Autodesk Inventor part; units mm, degrees
ref_plane "YZ Plane" through (0, 0, 0) normal (1, 0, 0) x (0, 1, 0)
ref_plane "XZ Plane" through (0, 0, 0) normal (0, 1, 0) x (-1, 0, 0)
ref_plane "XY Plane" through (0, 0, 0) normal (0, 0, 1) x (1, 0, 0)
sketch "Sketch2" plane through (0, 0, 0) normal (1, 0, 0) x (0, 1, 0)
  circle A0 centre (0, 0) radius 21.5
  dimension "d3" = 43
extrude "Extrusion1" add sketch "Sketch2" along normal blind 2
sketch "Sketch3" plane through (2, 0, 0) normal (1, 0, 0) x (0, 0, -1)
  circle A0 centre (0, 0) radius 21.5
  circle A1 centre (0, 0) radius 8.5
  dimension "d6" = 17
extrude "Extrusion2" cut sketch "Sketch3" against normal blind 2 contours A1
sketch "Sketch4" plane through (2, 0, 0) normal (1, 0, 0) x (0, 0, -1)
  circle A0 centre (0, 0) radius 8.5
  circle A1 centre (0, 0) radius 21.5
  circle A2 centre (0, 0) radius 9.5
  dimension "d9" = 19
extrude "Extrusion3" add sketch "Sketch4" along normal blind 7 contours A2
properties part number "holeCoverP2"
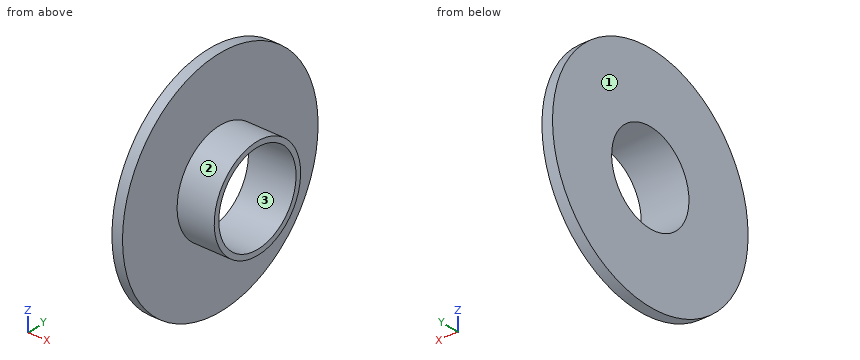
Read the model definition and answer for the solid it produces. Units are mm, in the model's axes. Face numbers are marked on the shaded views. Give positions to 0.01 mm unless a question says otherwise; leave off trailing zeros. Write each loop counter-clockwise with the first axis right and the second up, starting at its lowest first coordinate (ties: lowest second). Pieces come first, ordered by that corner, then holes. Notation, with made-up numbers: (50, -15) -> (87, -15) arc R35 ccw to (87, 20) -> close; hole circle Ø6 at (-4, -34). An arc over 180 degrees is marked (long way). Answer in a Markdown table with one row per item.
1) Straight lines are drawn through the part: line 1 (Y direction, x = 2.25, z = 0); line 2 (X direction, y = -10.5, z = 7); line 3 (Y direction, x = 6.5, z = 1). For each, find the intervals that lie inside material, in ascending order. Write a range as [from, to].
Results list:
| item | result |
|---|---|
| line 1 | [-9.5, -8.5], [8.5, 9.5] |
| line 2 | [0, 2] |
| line 3 | [-9.45, -8.44], [8.44, 9.45] |
2) Section D-D on z = -9 is taken. Give the vertices of the cut face in (x, y), plus the area to 3 significant figures.
Results list:
| item | result |
|---|---|
| outline | (0, -19.53) -> (2, -19.53) -> (2, -3.04) -> (9, -3.04) -> (9, 3.04) -> (2, 3.04) -> (2, 19.53) -> (0, 19.53) -> close |
| area | 121 mm^2 |
3) Each of these flat-tipped pins is pushed along its axis until it touches: pin 1 Ø1 at (x, z) = (3.5, 2) entering from +Y; pin 2 Ø13.5 at (y, z) = (0, 0) entering from -X; pin 3 Ø2 at (x, y) = (4, -6.5) entering from -Z; pin 4 Ø1.5 at (x, z) = (3.5, -9) entering from +Y. Where does it stop, or does it pass through?
Results list:
| item | result |
|---|---|
| pin 1 | y = 9.38 |
| pin 2 | through |
| pin 3 | z = -7.75 |
| pin 4 | y = 4.71 |
4) Determine the mould class of the marked faces 1, 2 and 3 for opening direction Y: released by +Y, released by -Y, zero draft, split by the parting line, or undercut.
Results list:
| item | result |
|---|---|
| face 1 | zero draft |
| face 2 | split by the parting line |
| face 3 | undercut |
5) Section C-C on x = 8 is taken. Give the vertices of the cut face in (y, z), plus the area to 3 significant figures.
Results list:
| item | result |
|---|---|
| outline | circle Ø19 at (0, 0); hole circle Ø17 at (0, 0) |
| area | 56.5 mm^2 |
6) Section A-A on z = 0 is taken. Give the vertices of the cut face in (x, y).
Results list:
| item | result |
|---|---|
| outline | (0, -21.5) -> (2, -21.5) -> (2, -9.5) -> (9, -9.5) -> (9, -8.5) -> (0, -8.5) -> close; (0, 8.5) -> (9, 8.5) -> (9, 9.5) -> (2, 9.5) -> (2, 21.5) -> (0, 21.5) -> close |
